Verification items for the finished model (mm, model axes). A direction names the side the tool comes from. Coordinates: 2 decimals unless noted, no trailing zeros. Write each loop counter-clockwise with the first axis right and the second up, starting at its lowest first coordinate (ties: lowest second). Pieces come first, ordered by that corner, then holes. Notation, with made-up numbers: (-24, 51) -> (-16, 51) arc R6 ccw to (-16, 58) -> close; hole circle Ø8 at (45.5, 5). An arc over 180 degrees is marked (long way). Answer in a Markdown table with one row per item.
```python
from build123d import *

# Parameters (mm, degrees)
ESQUISSE1_R             = 25
BOSS_EXTRU_1_DEPTH      = 30
ESQUISSE2_R             = 4
BOSS_EXTRU_2_DEPTH      = 39
ESQUISSE3_R             = 5
BOSS_EXTRU_3_DEPTH      = 1
ESQUISSE4_R             = 3
ENL_V_MAT_EXTRU_1_DEPTH = 10
CHANFREIN1_SIZE         = 0.5
ESQUISSE5_W             = 10
ESQUISSE5_H             = 1


with BuildPart() as part:
    # Esquisse1 → Boss.-Extru.1 (new body)
    with BuildSketch(Plane.XY):
        Circle(ESQUISSE1_R)
    extrude(amount=BOSS_EXTRU_1_DEPTH)

    # Esquisse2 → Boss.-Extru.2 (add)
    with BuildSketch(Plane.XY.offset(30)):
        Circle(ESQUISSE2_R)
    extrude(amount=BOSS_EXTRU_2_DEPTH)

    # Esquisse3 → Boss.-Extru.3 (add)
    with BuildSketch(Plane.XY.offset(30)):
        Circle(ESQUISSE3_R)
    extrude(amount=BOSS_EXTRU_3_DEPTH)

    # Esquisse4 → Enlèv. mat.-Extru.1 (cut)
    with BuildSketch(Plane(origin=(0, 0, 0), x_dir=(-1, 0, 0), z_dir=(0, 0, -1))):
        Circle(ESQUISSE4_R)
    extrude(amount=-ENL_V_MAT_EXTRU_1_DEPTH, mode=Mode.SUBTRACT)

    # Chanfrein1
    chanfrein1_edges = [part.edges().sort_by_distance(p)[0] for p in [
        (-25, 0, 0),
        (-25, 0, 30),
        (-4, 0, 69),
    ]]
    chamfer(chanfrein1_edges, length=CHANFREIN1_SIZE)

    # Esquisse5 → Enlèvement de matière-Révolution1 (revolve, cut)
    with BuildSketch(Plane(origin=(0, 0, 0), x_dir=(0, 0, -1), z_dir=(1, 0, 0)), mode=Mode.PRIVATE) as enl_vement_de_mati_re_r_volution1_sk:
        with Locations((-64, 3.5)):
            Rectangle(ESQUISSE5_W, ESQUISSE5_H)
    revolve(enl_vement_de_mati_re_r_volution1_sk.sketch.rotate(Axis((0, 0, 69), (0, 0, -1)), 180), axis=Axis((0, 0, 69), (0, 0, -1)), mode=Mode.SUBTRACT)


solid = part.part
```
1. Section check D-D, the plane z = 53. Record the boundary of the cut face in (x, y).
Geometry says:
| item | result |
|---|---|
| outline | circle Ø8 at (0, 0) |
2. Section check C-C, the plane z = 21. Record the boundary of the cut face in (x, y).
Geometry says:
| item | result |
|---|---|
| outline | circle Ø50 at (0, 0) |
3. Mould release check, pull along Y, two halves, no side actions. Record for faces 1 (the flat face through (5, 0, 0)), 2 (the cylindrical face through (3, 0, 5)), 3 (the cylindrical face through (3.815, 1.201, 44.804)): released by +Y, released by -Y, zero draft, split by the parting line, or undercut.
Geometry says:
| item | result |
|---|---|
| face 1 | zero draft |
| face 2 | undercut |
| face 3 | split by the parting line |
4. Depth check by flat-ended pin: P1, Ø5, axis at x = -0.5, y = 1.5, coming from the -Z side; P2, Ø2, axis at x = -17.5, z = 31.5, coming from the +Y side; P3, Ø1.5, axis at x = -1, z = 46.5, coming from the -Y side; P4, Ø1, axis at x = -3.5, y = 6, coming from the +Z side. Enter the tip coordinate at first touch or a pass-through.
Geometry says:
| item | result |
|---|---|
| P1 | z = 0 |
| P2 | through |
| P3 | y = -3.99 |
| P4 | z = 30 |
5. Section check A-A, the plane x = 0. Record the boundary of the cut face in (y, z).
Geometry says:
| item | result |
|---|---|
| outline | (-25, 0.5) -> (-24.5, 0) -> (-3, 0) -> (-3, 10) -> (3, 10) -> (3, 0) -> (24.5, 0) -> (25, 0.5) -> (25, 29.5) -> (24.5, 30) -> (5, 30) -> (5, 31) -> (4, 31) -> (4, 59) -> (3, 59) -> (3, 69) -> (-3, 69) -> (-3, 59) -> (-4, 59) -> (-4, 31) -> (-5, 31) -> (-5, 30) -> (-24.5, 30) -> (-25, 29.5) -> close |
6. Tool access check on faces 4 (the flat face through (0, 0, 10)), 5 (the flat face through (-3, 1, 59)), 6 (the flat face through (0, 0, 69)). Record the directions out of +Z, -Z, +X, -X, +Y, -Y that give a thin tool (end or side, any length) a straight path to the whole face; none if there is none.
Geometry says:
| item | result |
|---|---|
| face 4 | -Z |
| face 5 | +Z |
| face 6 | +Z, +X, -X, +Y, -Y |
7. Thickness scan on line 1 (Y direction, x = 0, z = 2.5); line 2 (Z direction, x = -18.5, y = 8.5); line 3 (X direction, y = 16.5, z = 19.5). Record the ranges inside material, lowest first. Write a range as from..to.
Geometry says:
| item | result |
|---|---|
| line 1 | -25..-3, 3..25 |
| line 2 | 0..30 |
| line 3 | -18.78..18.78 |
